The figure shows three views and two pictorial views of one solid part (mm, origin at its lowest corner). Answer the questions. A direction names the side the tool comes from. Give positions to 0.01 mm unless a question says otherwise; leave off trailing zeros. Order: outer loops, then holes, each group sorted by start corner. A loop starts at its lowest first (then second) coordinate and runs counter-clockwise, first axis right, second up. Notation, with made-up numbers: (-36.5, 28.5) -> (15.5, 28.5) arc R14 cw to (15.5, 39.5) -> close; hole circle Ø5 at (71, 49). An arc over 180 degrees is marked (long way). Use one line per item in the form item = value.
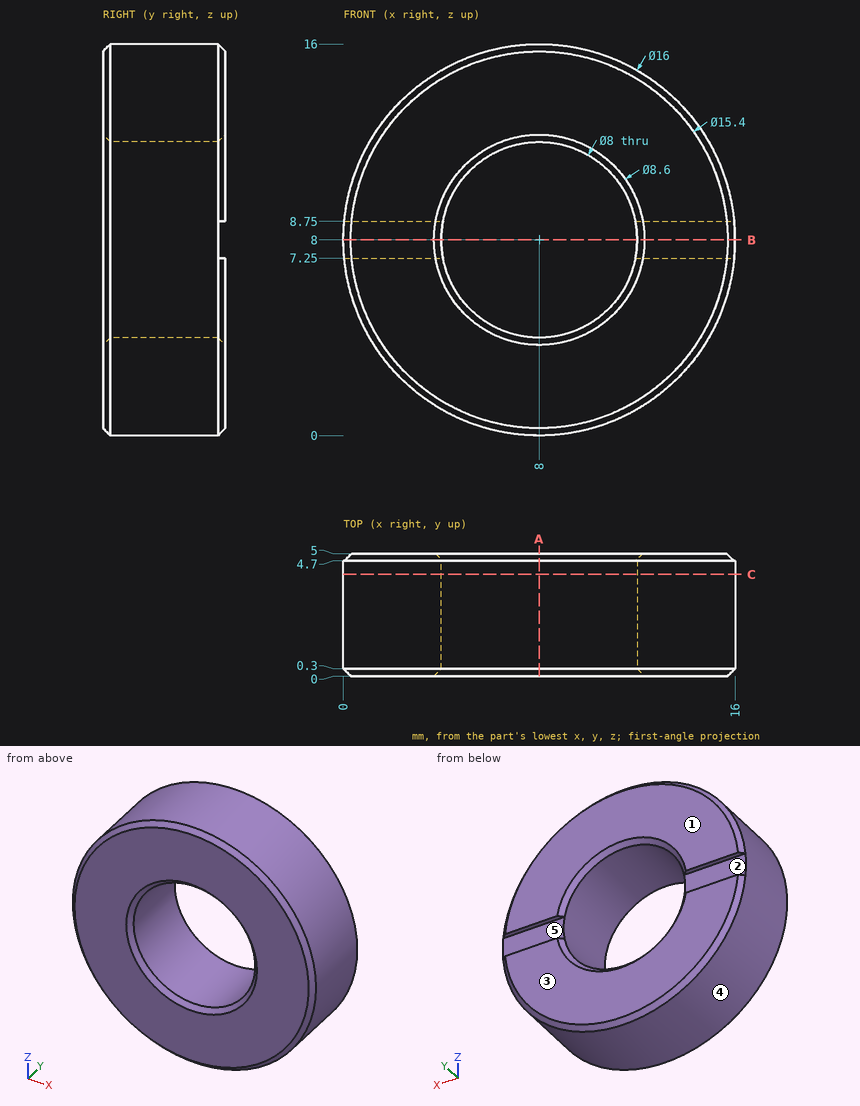
Item 1: The part is cut by section A-A on x = 8. Give the vertices of the cut face in (y, z).
Checks:
outline = (0, 0.3) -> (0.3, 0) -> (4.7, 0) -> (5, 0.3) -> (5, 3.7) -> (4.7, 4) -> (0.3, 4) -> (0, 3.7) -> close; (0, 12.3) -> (0.3, 12) -> (4.7, 12) -> (5, 12.3) -> (5, 15.7) -> (4.7, 16) -> (0.3, 16) -> (0, 15.7) -> close
Item 2: The part is cut by section C-C on y = 4.15. Give the vertices of the cut face in (x, z).
Checks:
outline = circle Ø16 at (8, 8); hole circle Ø8 at (8, 8)
Item 3: Straight lines are drawn through the part: L1, parallel to Z at x = 8, y = 3.8; L2, parallel to Z at x = 4.75, y = 1.6; L3, parallel to X at y = 2.5, z = 7. For each, find the intervals that lie inside material, in ascending order. Write a range as from..to.
Checks:
L1 = 0..4, 12..16
L2 = 0.69..5.67, 10.33..15.31
L3 = 0.06..4.13, 11.87..15.94
Item 4: The part is cut by section B-B on z = 8. Give the vertices of the cut face in (x, y).
Checks:
outline = (0, 0.3) -> (0.3, 0) -> (3.7, 0) -> (4, 0.3) -> (4, 4.7) -> (0, 4.7) -> close; (12, 0.3) -> (12.3, 0) -> (15.7, 0) -> (16, 0.3) -> (16, 4.7) -> (12, 4.7) -> close
Item 5: Given pin 1 Ø5 at (x, z) = (8, 8) entering from +Y; pin 2 Ø1.7 at (x, z) = (3, 8.5) entering from +Y; pin 3 Ø1 at (x, y) = (3.5, 2) entering from -Z; pin 4 Ø1.5 at (x, y) = (4, 2) entering from +Z, each flat-ended and moving along its own axis, determine where each tip first touches the part or whether it passes through.
Checks:
pin_1 = through
pin_2 = 5
pin_3 = 1.07
pin_4 = 15.31
Item 6: Which of the six approach directions +Z, -Z, +X, -X, +Y, -Y give full straight-line access (tool end or side, diameter ignored) to the marked faces 1 and 2?
Checks:
face_1 = +Z, -Z, +X, -X, +Y
face_2 = +X, -X, +Y
Item 7: Determine the mould class of the marked faces 3, 4 and 5 for opening direction Z: +Z half, -Z half, draft (parallel to the pull), parting line (faces both ways), or undercut.
Checks:
face_3 = draft
face_4 = parting line
face_5 = undercut
